The figure shows three views and two pictorial views of one solid part (mm, origin at its lowest corner). Answer the questions. A direction names the side the tool comes from. Give positions to 0.01 mm unless a question says otherwise; leave off trailing zeros. Loops run counter-clockwise (first coordinate to the right, second up) from the corner with the lowest first, then second, coordinate; pieces in that order, holes last. Notation, with made-up numbers: (-33.75, 23.5) - (4.25, 23.5) arc R22 cw to (4.25, 49.5) - close; hole circle Ø4 at (22, 40). An arc over 180 degrees is marked (long way). Use a Markdown table: item, result. Add a question column.
Item 1: Consider probe 1 along Y at (x, z) = (103, 10) (1 decimal); probe 2 along Y at (x, z) = (56.5, 30) (1 decimal); probe 3 along X at (y, z) = (17.5, 17). Determine where each line is inside the solid, lowest interval first. Write a range as [from, to].
Item 2: Which of the six approach directions +Z, -Z, +X, -X, +Y, -Y give full straight-line access (tool end or side, diameter ignored) to the marked faces 5, 6 and 7?
Item 3: A cutting plane is placed at D-D (x = 69.5). Determine the outline of the cut face in (y, z) (1 decimal).
Item 4: Each of these flat-tipped pins is pushed along its axis until it touches: P1, Ø6.5, axis at x = 45.5, z = 14, coming from the +Y side; P2, Ø1, axis at y = 52.5, z = 33, coming from the -X side (1 decimal); P3, Ø2, axis at y = 15.5, z = 19.5, coming from the -X side; P4, Ø2, axis at x = 51, z = 32, coming from the +Y side (1 decimal). Where does it stop, or does it pass through?
Item 5: A cutting plane is placed at C-C (x = 105.5). Determine the outline of the cut face in (y, z).
Item 6: A cutting plane is placed at B-B (y = 47.5). Determine the outline of the cut face in (x, z).
Item 7: For a pull along X with two mould halves and no side action, classify the marked faces 1, 2, 3 and 4 as +X half, -X half, draft (parallel to the pull), parting line (faces both ways), or undercut.
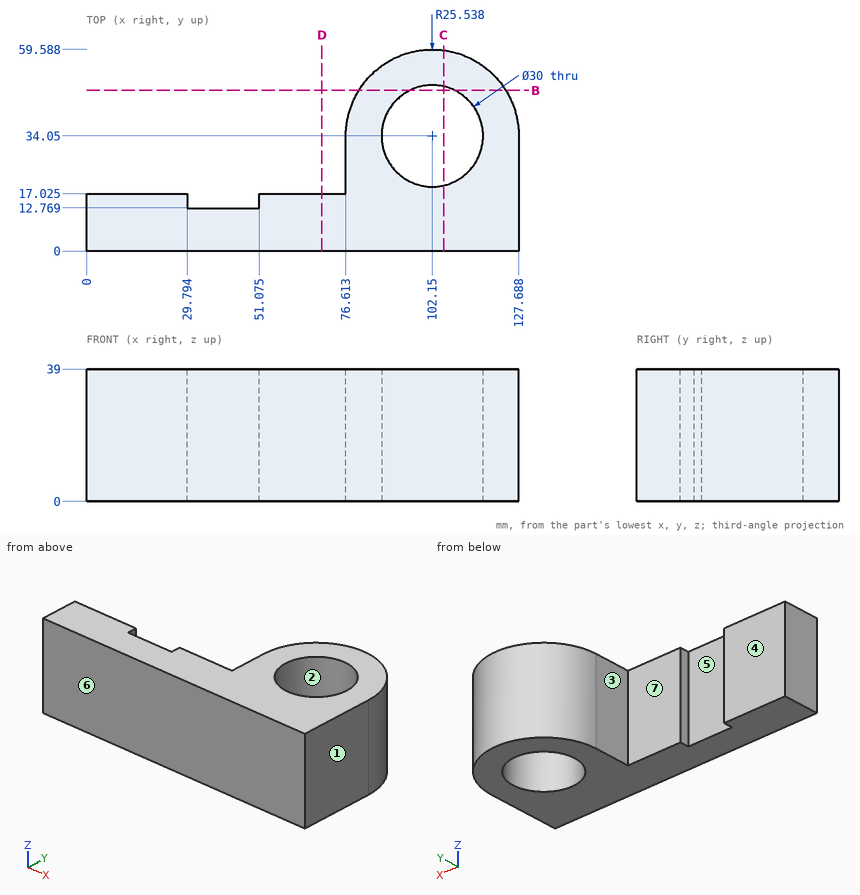
Geometry says:
| question | item | result |
|---|---|---|
| 1 | probe 1 | [0, 19.1], [49, 59.6] |
| 1 | probe 2 | [0, 17] |
| 1 | probe 3 | [76.61, 127.69] |
| 2 | face 5 | +Z, -Z, +Y |
| 2 | face 6 | +Z, -Z, +X, -X, -Y |
| 2 | face 7 | +Z, -Z, -X, +Y |
| 3 | outline | (0, 0) - (17, 0) - (17, 39) - (0, 39) - close |
| 4 | P1 | y = 12.77 |
| 4 | P2 | x = 84 |
| 4 | P3 | x = 0 |
| 4 | P4 | y = 17 |
| 5 | outline | (0, 0) - (19.43, 0) - (19.43, 39) - (0, 39) - close; (48.67, 0) - (59.37, 0) - (59.37, 39) - (48.67, 39) - close |
| 6 | outline | (80.44, 0) - (95.51, 0) - (95.51, 39) - (80.44, 39) - close; (108.79, 0) - (123.86, 0) - (123.86, 39) - (108.79, 39) - close |
| 7 | face 1 | +X half |
| 7 | face 2 | undercut |
| 7 | face 3 | -X half |
| 7 | face 4 | draft |
